Check sheet for the modelled part. Datum: model origin and axes. Units: mm. A direction names the side the tool comes from. Round coordinates to 2 decimals unless told otherwise and drop trailing zeros. Loops run counter-clockwise (first coordinate to the right, second up) from the corner with the lowest first, then second, coordinate; pieces in that order, holes last. Notation, with made-up numbers: (46.25, 7.25) - (82.25, 7.25) arc R20 ccw to (82.25, 12.25) - close; hole circle Ø4 at (88.25, 14.25). An arc over 180 degrees is marked (long way). Answer in a Markdown table with one row per item. Add a question column.
(1) Thickness scan on line 1 along Z through (x, y) = (33, 0.85); line 2 along X through (y, z) = (2.05, 22.75); line 3 along Z through (x, y) = (-15.5, 0.8). Record the ranges inside material, lowest first.
(2) Cross-section at B-B on x = -12. Enter the section's corners in (y, z), then the cut area to 3 significant figures.
(3) Cross-section at A-A on z = 22.75. Enter the section's corners in (x, y).
(4) Mould release check, pull along Z, two halves, no side actions. Record for faces 3 (the flat face through (8, 0, 23)), 4 (the flat face through (0, 1, -23.75)), 5 (the flat face through (-34, 1, 0)): +Z half, -Z half, draft (parallel to the pull), parting line (faces both ways), or undercut.
(5) Gauge pin test, flat ends, axial feed: pin 1 (1.5 mm diameter, centred on y = 1, z = -5, fed in from +X); pin 2 (1.5 mm diameter, centred on x = -11, y = 1.5, fed in from -Z); pin 3 (1.2 mm diameter, centred on x = 33, z = -22.75, fed in from +Y); pin 4 (1.5 mm diameter, centred on y = 1, z = -3, fed in from -X). Record the tip position at first contact, or that the pin passes through.
(6) Cross-section at D-D on x = 33. Enter the section's corners in (y, z), then the cut area to 4 significant figures.
(7) Cross-section at C-C on z = 9. Enter the section's corners in (x, y).
(8) Access from +Z, -Z, +X, -X, +Y, -Y to the whole of each face (thin tool, end or side, straight path). Record for faces 1 (the flat face through (0, 1, -21.75)), 2 (the flat face through (34, 1, 0)).
Autodesk Inventor part; units mm, degrees
ref_plane "YZ Plane" through (0, 0, 0) normal (1, 0, 0) x (0, 1, 0)
ref_plane "XZ Plane" through (0, 0, 0) normal (0, 1, 0) x (-1, 0, 0)
ref_plane "XY Plane" through (0, 0, 0) normal (0, 0, 1) x (1, 0, 0)
sketch "Sketch1" plane through (0, 0, 0) normal (0, 1, 0) x (-1, 0, 0)
  line L0 (-33, 22.75) -> (33, 22.75) construction
  line L1 (33, 22.75) -> (33, -22.75) construction
  line L2 (33, -22.75) -> (-33, -22.75) construction
  line L3 (-33, -22.75) -> (-33, 22.75) construction
  line L4 (-33, 22.75) -> (33, -22.75) construction
  line L5 (33, 22.75) -> (-33, -22.75) construction
  line L6 (32, -21.75) -> (32, 21.75)
  line L7 (32, 21.75) -> (-32, 21.75)
  line L8 (-32, 21.75) -> (-32, -21.75)
  line L9 (-32, -21.75) -> (32, -21.75)
  line L10 (34, -23.75) -> (34, 23.75)
  line L11 (34, 23.75) -> (-34, 23.75)
  line L12 (-34, 23.75) -> (-34, -23.75)
  line L13 (-34, -23.75) -> (34, -23.75)
  point P0 (0, 0)
  dimension "d0" = 45.5
  dimension "d1" = 66
  dimension "d18" = 1
  dimension "d19" = 1
extrude "Extrusion1" add sketch "Sketch1" along normal blind 3
sketch "Sketch4" plane through (0, 3, 0) normal (0, 1, 0) x (1, 0, 0)
  line L0 (-32, -21.75) -> (-32, 21.75) construction
  line L1 (-34, 23.75) -> (-32, 21.75) construction
  line L2 (33, -22.75) -> (-33, -22.75) construction
  line L3 (-33, -22.75) -> (-33, 22.75) construction
  line L4 (-33, 22.75) -> (33, 22.75) construction
  line L5 (33, 22.75) -> (33, -22.75) construction
  line L6 (33, -22.75) -> (-33, 22.75) construction
  line L7 (-33, -22.75) -> (33, 22.75) construction
  circle A0 centre (-33, 22.75) radius 3
  circle A1 centre (33, 22.75) radius 3
  circle A2 centre (-33, -22.75) radius 3
  circle A3 centre (33, -22.75) radius 3
  point P0 (0, 0)
  dimension "d20" = 6
  dimension "d21" = 6
  dimension "d22" = 6
  dimension "d23" = 6
extrude "Extrusion3" add sketch "Sketch4" against normal up to surface (3 mm away)
sketch "Sketch5" plane through (0, 3, 0) normal (0, 1, 0) x (1, 0, 0)
  line L0 (-30.1716, -23.75) -> (30.1716, -23.75)
  arc A0 (30.1716, -23.75) -> (34, -19.9216) centre (33, -22.75) ccw
  line L1 (34, -19.9216) -> (34, 19.9216)
  arc A1 (34, 19.9216) -> (30.1716, 23.75) centre (33, 22.75) ccw
  line L2 (30.1716, 23.75) -> (-30.1716, 23.75)
  arc A2 (-30.1716, 23.75) -> (-34, 19.9216) centre (-33, 22.75) ccw
  line L3 (-34, 19.9216) -> (-34, -19.9216)
  arc A3 (-34, -19.9216) -> (-30.1716, -23.75) centre (-33, -22.75) ccw
  arc A4 (-30.1716, -21.75) -> (-32, -19.9216) centre (-33, -22.75) ccw
  line L4 (-32, -19.9216) -> (-32, 19.9216)
  arc A5 (-32, 19.9216) -> (-30.1716, 21.75) centre (-33, 22.75) ccw
  line L5 (-30.1716, 21.75) -> (30.1716, 21.75)
  arc A6 (30.1716, 21.75) -> (32, 19.9216) centre (33, 22.75) ccw
  line L6 (32, 19.9216) -> (32, -19.9216)
  arc A7 (32, -19.9216) -> (30.1716, -21.75) centre (33, -22.75) ccw
  line L7 (30.1716, -21.75) -> (-30.1716, -21.75)
  point P0 (0, 0)
hole "Hole2" at (-33, 3, -22.75) at (33, 3, -22.75) at (-33, 3, 22.75) at (33, 3, 22.75) direction (0, -1, 0) diameter 2 depth 25 tip angle 118
equation "\"d18\" = d19"
equation "\"d21\" = d20"
equation "\"d22\" = d20"
equation "\"d23\" = d20"
properties part number "soporte_placa_separador"
Answers:
| question | item | result |
|---|---|---|
| 1 | line 1 | z = -25.75 to -23.75, -21.75 to 21.75, 23.75 to 25.75 |
| 1 | line 2 | x = -36 to -34, -32 to 32, 34 to 36 |
| 1 | line 3 | z = -23.75 to -21.75, 21.75 to 23.75 |
| 2 | outline | (0, -23.75) - (3, -23.75) - (3, -21.75) - (0, -21.75) - close; (0, 21.75) - (3, 21.75) - (3, 23.75) - (0, 23.75) - close |
| 2 | area | 12.0 mm^2 |
| 3 | outline | (-36, 0) - (-34, 0) - (-34, 3) - (-36, 3) - close; (-32, 0) - (32, 0) - (32, 3) - (-32, 3) - close; (34, 0) - (36, 0) - (36, 3) - (34, 3) - close |
| 4 | face 3 | draft |
| 4 | face 4 | -Z half |
| 4 | face 5 | undercut |
| 5 | pin 1 | stops at x = 34 |
| 5 | pin 2 | stops at z = -23.75 |
| 5 | pin 3 | passes through |
| 5 | pin 4 | stops at x = -34 |
| 6 | outline | (0, -25.75) - (3, -25.75) - (3, -23.75) - (0, -23.75) - close; (0, -21.75) - (3, -21.75) - (3, 21.75) - (0, 21.75) - close; (0, 23.75) - (3, 23.75) - (3, 25.75) - (0, 25.75) - close |
| 6 | area | 142.5 mm^2 |
| 7 | outline | (-34, 0) - (-32, 0) - (-32, 3) - (-34, 3) - close; (32, 0) - (34, 0) - (34, 3) - (32, 3) - close |
| 8 | face 1 | +Y, -Y |
| 8 | face 2 | +X, +Y, -Y |
